Check sheet for the modelled part. Datum: model origin and axes. Units: mm. Face numbers are marked on the shaded views. A direction names the side the tool comes from. Round coordinates to 2 decimals unless told otherwise and drop trailing zeros. Order: outer loops, then holes, each group sorted by start corner. A loop starts at its lowest first (then second) coordinate and runs counter-clockwise, first axis right, second up.
Q1. Depth check by flat-ended pin: P1, Ø3, axis at y = 28, z = 20.5, coming from the -X side; P2, Ø10.5, axis at x = 70, z = 14, coming from the -Y side; P3, Ø3, axis at y = 38, z = 12.5, coming from the +X side; P4, Ø8.5, axis at x = 43.5, z = 15, coming from the +Y side. Enter the tip coordinate at first touch or a pass-through.
Q2. Cross-section at D-D on y = 24. Record the cut outline in (x, z).
Q3. Cross-section at A-A on z = 5.25. Record the cut outline in (x, y).
Q4. Cross-section at C-C on z = 14. Record the cut outline in (x, y).
Q5. Set-up check for the marked faces 5, 6 and 7: record each of +Z, -Z, +X, -X, +Y, -Y from which the full face is reachable in a straight line by a thin tool's end or side.
Q6. Scan lines: probe 1 along X at (y, z) = (5, 14); probe 2 along X at (y, z) = (5.75, 14); probe 3 along Y at (x, z) = (56, 25.75). Record each from-to range of solid material in increasing order.
Q7. Mould release check, pull along X, two halves, no side actions. Record for the marked faces 1, 2, 3 and 4: +X half, -X half, draft (parallel to the pull), parting line (faces both ways), or undercut.
Q8. Cross-section at B-B on x = 70. Record the cut outline in (y, z), then the cut area to 3 significant figures.
from build123d import *

# Parameters (mm, degrees)
EXTRUDE_1_DEPTH     = 28
SKETCH_3_R          = 3.25
CUT_EXTRUDE_1_DEPTH = 10
SKETCH_4_R          = 3.25
CUT_EXTRUDE_2_DEPTH = 10


with BuildPart() as part:
    # 草图2 → 凸台-拉伸1 (new body)
    with BuildSketch(Plane.XY):
        Polygon((56.568542495, 56.568542495), (0, 0), (80, 0), (80, 8), (60, 8), (48.083261121, 36.769552622), (62.225396744, 50.911688245), align=None)
        Polygon((7.242640687, 3), (43.716092715, 39.473452028), (58.823891211, 3), align=None, mode=Mode.SUBTRACT)
    extrude(amount=EXTRUDE_1_DEPTH)

    # 草图3 → 切除-拉伸1 (cut)
    with BuildSketch(Plane(origin=(0, 8, 0), x_dir=(1, 0, 0), z_dir=(0, 1, 0))):
        with Locations(Location((70, -14, 0), (0, 0, 270))):
            Circle(SKETCH_3_R)
    extrude(amount=-CUT_EXTRUDE_1_DEPTH, mode=Mode.SUBTRACT)

    # 草图4 → 切除-拉伸2 (cut)
    with BuildSketch(Plane(origin=(5.656854249, -5.656854249, 0), x_dir=(0, 0, -1), z_dir=(0.7071067811865439, -0.7071067811865511, 0))):
        with Locations(Location((-14, 70, 0), (0, 0, 90))):
            Circle(SKETCH_4_R)
    extrude(amount=-CUT_EXTRUDE_2_DEPTH, mode=Mode.SUBTRACT)


solid = part.part
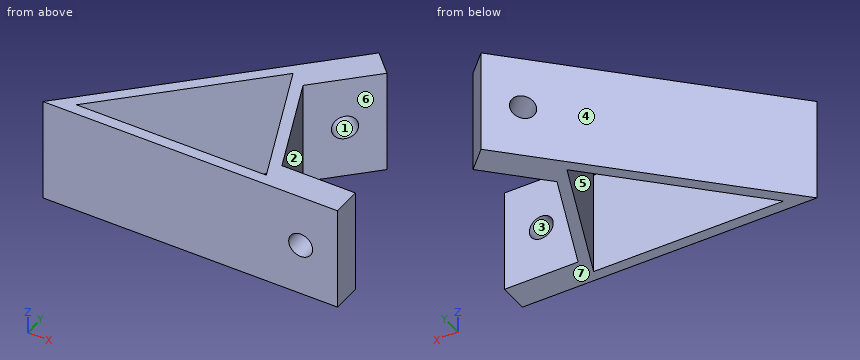
Results found:
1. P1: stops at x = 26.5
1. P2: stops at y = 0
1. P3: stops at x = 50.81
1. P4: stops at y = 47.65
2. outline: (24, 0) - (28.24, 0) - (28.24, 28) - (24, 28) - close; (50.13, 0) - (53.37, 0) - (53.37, 28) - (50.13, 28) - close
3. outline: (0, 0) - (80, 0) - (80, 8) - (60, 8) - (48.08, 36.77) - (62.23, 50.91) - (56.57, 56.57) - close; hole (7.24, 3) - (58.82, 3) - (43.72, 39.47) - close
4. outline: (0, 0) - (66.75, 0) - (66.75, 8) - (60, 8) - (48.08, 36.77) - (52.86, 41.54) - (47.2, 47.2) - close; (51.8, 51.8) - (57.45, 46.14) - (62.23, 50.91) - (56.57, 56.57) - close; (73.25, 0) - (80, 0) - (80, 8) - (73.25, 8) - close; hole (7.24, 3) - (58.82, 3) - (43.72, 39.47) - close
5. face 5: +Z, -Z
5. face 6: +Z, -Z, +X
5. face 7: -Z, +X, -X, +Y, -Y
6. probe 1: x = 5 to 9.24, 58 to 66.75, 73.25 to 80
6. probe 2: x = 5.75 to 9.99, 57.68 to 66.75, 73.25 to 80
6. probe 3: y = 0 to 3, 9.82 to 17.66, 44.69 to 56
7. face 1: undercut
7. face 2: +X half
7. face 3: undercut
7. face 4: -X half
8. outline: (0, 0) - (8, 0) - (8, 10.75) - (0, 10.75) - close; (0, 17.25) - (8, 17.25) - (8, 28) - (0, 28) - close
8. area: 172 mm2
